```python
from build123d import *

# Parameters (mm, degrees)
EXTRUDE_1_DEPTH     = 6
EXTRUDE_2_DEPTH     = 20
EXTRUDE_4_DEPTH     = 6
SKETCH_5_R          = 7.25
EXTRUDE_5_DEPTH     = 14.8
SKETCH_6_R          = 4.25
SKETCH_6_R_2        = 1.25
EXTRUDE_6_DEPTH     = 10.2
EXTRUDE_7_DEPTH     = 76
CUT_EXTRUDE_1_DEPTH = 76


with BuildPart() as part:
    # 草图1 → 凸台-拉伸1 (new body)
    with BuildSketch(Plane(origin=(0, 0, 0), x_dir=(1, 0, 0), z_dir=(0, 1, 0))):
        with BuildLine():
            Line((-5, 0), (-5, -18))
            Line((-5, -18), (15, -18))
            Line((15, -18), (15, -88))
            Line((15, -88), (-10, -88))
            Line((-10, -88), (-10, -91))
            Line((-10, -91), (18, -91))
            Line((18, -91), (18, -15))
            Line((18, -15), (5, -15))
            Line((5, -15), (5, 0))
            ThreePointArc((5, 0), (0, 5), (-5, 0))
        make_face()
    extrude(amount=-EXTRUDE_1_DEPTH)

    # 草图2 → 凸台-拉伸2 (add, symmetric)
    with BuildSketch(Plane(origin=(0, 0, 0), x_dir=(1, 0, 0), z_dir=(0, 1, 0))):
        Polygon((-5, -18), (15, -18), (15, -88), (-10, -88), (-10, -91), (18, -91), (18, -15), (-5, -15), align=None)
    extrude(amount=EXTRUDE_2_DEPTH, both=True)

    # 草图4 → 凸台-拉伸4 (add)
    with BuildSketch(Plane.XZ.offset(6)):
        with BuildLine():
            ThreePointArc((-0.504732798, 8.734428762), (-0.823506466, 9.891100464), (-1.470958285, 10.901205517))
            ThreePointArc((-1.470958285, 10.901205517), (-1.726760313, 10.86362273), (-1.981608382, 10.820038273))
            ThreePointArc((-1.981608382, 10.820038273), (-2.283953757, 9.65896405), (-2.228374617, 8.460457882))
            ThreePointArc((-2.228374617, 8.460457882), (-2.708170263, 8.319303747), (-3.17911634, 8.150964378))
            ThreePointArc((-3.17911634, 8.150964378), (-3.839719327, 9.152518056), (-4.767622226, 9.913111434))
            ThreePointArc((-4.767622226, 9.913111434), (-4.999290692, 9.798320906), (-5.228197271, 9.678117239))
            ThreePointArc((-5.228197271, 9.678117239), (-5.156953143, 8.480440175), (-4.733735466, 7.357767973))
            ThreePointArc((-4.733735466, 7.357767973), (-5.146429214, 7.075257405), (-5.542305825, 6.76962681))
            ThreePointArc((-5.542305825, 6.76962681), (-6.480073708, 7.518023412), (-7.597598086, 7.954652936))
            ThreePointArc((-7.597598086, 7.954652936), (-7.782455665, 7.773891163), (-7.963013783, 7.588834659))
            ThreePointArc((-7.963013783, 7.588834659), (-7.525154025, 6.471791729), (-6.775725305, 5.53484847))
            ThreePointArc((-6.775725305, 5.53484847), (-7.080919818, 5.138635571), (-7.3629758, 4.725631002))
            ThreePointArc((-7.3629758, 4.725631002), (-8.486113324, 5.147612255), (-9.683868109, 5.217537585))
            ThreePointArc((-9.683868109, 5.217537585), (-9.803819655, 4.988498789), (-9.918355025, 4.756704069))
            ThreePointArc((-9.918355025, 4.756704069), (-9.1567404, 3.829639217), (-8.154459943, 3.170139435))
            ThreePointArc((-8.154459943, 3.170139435), (-8.322280653, 2.699008286), (-8.462906403, 2.219057507))
            ThreePointArc((-8.462906403, 2.219057507), (-9.661473042, 2.273316945), (-10.82221365, 1.969693302))
            ThreePointArc((-10.82221365, 1.969693302), (-10.86551747, 1.714797397), (-10.902818572, 1.458954141))
            ThreePointArc((-10.902818572, 1.458954141), (-9.892001226, 0.812614936), (-8.734979226, 0.495115065))
            ThreePointArc((-8.734979226, 0.495115065), (-8.748998674, -0.004816736), (-8.734428762, -0.504732798))
            ThreePointArc((-8.734428762, -0.504732798), (-9.891100464, -0.823506466), (-10.901205517, -1.470958285))
            ThreePointArc((-10.901205517, -1.470958285), (-10.86362273, -1.726760313), (-10.820038273, -1.981608382))
            ThreePointArc((-10.820038273, -1.981608382), (-9.65896405, -2.283953757), (-8.460457882, -2.228374617))
            ThreePointArc((-8.460457882, -2.228374617), (-8.319303747, -2.708170263), (-8.150964378, -3.17911634))
            ThreePointArc((-8.150964378, -3.17911634), (-9.152518056, -3.839719327), (-9.913111434, -4.767622226))
            ThreePointArc((-9.913111434, -4.767622226), (-9.798320906, -4.999290692), (-9.678117239, -5.228197271))
            ThreePointArc((-9.678117239, -5.228197271), (-8.480440175, -5.156953143), (-7.357767973, -4.733735466))
            ThreePointArc((-7.357767973, -4.733735466), (-7.075257405, -5.146429214), (-6.76962681, -5.542305825))
            ThreePointArc((-6.76962681, -5.542305825), (-7.518023412, -6.480073708), (-7.954652936, -7.597598086))
            ThreePointArc((-7.954652936, -7.597598086), (-7.773891163, -7.782455665), (-7.588834659, -7.963013783))
            ThreePointArc((-7.588834659, -7.963013783), (-6.471791729, -7.525154025), (-5.53484847, -6.775725305))
            ThreePointArc((-5.53484847, -6.775725305), (-5.138635571, -7.080919818), (-4.725631002, -7.3629758))
            ThreePointArc((-4.725631002, -7.3629758), (-5.147612255, -8.486113324), (-5.217537585, -9.683868109))
            ThreePointArc((-5.217537585, -9.683868109), (-4.988498789, -9.803819655), (-4.756704069, -9.918355025))
            ThreePointArc((-4.756704069, -9.918355025), (-3.829639217, -9.1567404), (-3.170139435, -8.154459943))
            ThreePointArc((-3.170139435, -8.154459943), (-2.699008286, -8.322280653), (-2.219057507, -8.462906403))
            ThreePointArc((-2.219057507, -8.462906403), (-2.273316945, -9.661473042), (-1.969693302, -10.82221365))
            ThreePointArc((-1.969693302, -10.82221365), (-1.714797397, -10.86551747), (-1.458954141, -10.902818572))
            ThreePointArc((-1.458954141, -10.902818572), (-0.812614936, -9.892001226), (-0.495115065, -8.734979226))
            ThreePointArc((-0.495115065, -8.734979226), (0.004816736, -8.748998674), (0.504732798, -8.734428762))
            ThreePointArc((0.504732798, -8.734428762), (0.823506466, -9.891100464), (1.470958285, -10.901205517))
            ThreePointArc((1.470958285, -10.901205517), (1.726760313, -10.86362273), (1.981608382, -10.820038273))
            ThreePointArc((1.981608382, -10.820038273), (2.283953757, -9.65896405), (2.228374617, -8.460457882))
            ThreePointArc((2.228374617, -8.460457882), (2.708170263, -8.319303747), (3.17911634, -8.150964378))
            ThreePointArc((3.17911634, -8.150964378), (3.839719327, -9.152518056), (4.767622226, -9.913111434))
            ThreePointArc((4.767622226, -9.913111434), (4.999290692, -9.798320906), (5.228197271, -9.678117239))
            ThreePointArc((5.228197271, -9.678117239), (5.156953143, -8.480440175), (4.733735466, -7.357767973))
            ThreePointArc((4.733735466, -7.357767973), (5.146429214, -7.075257405), (5.542305825, -6.76962681))
            ThreePointArc((5.542305825, -6.76962681), (6.480073708, -7.518023412), (7.597598086, -7.954652936))
            ThreePointArc((7.597598086, -7.954652936), (7.782455665, -7.773891163), (7.963013783, -7.588834659))
            ThreePointArc((7.963013783, -7.588834659), (7.525154025, -6.471791729), (6.775725305, -5.53484847))
            ThreePointArc((6.775725305, -5.53484847), (7.080919818, -5.138635571), (7.3629758, -4.725631002))
            ThreePointArc((7.3629758, -4.725631002), (8.486113324, -5.147612255), (9.683868109, -5.217537585))
            ThreePointArc((9.683868109, -5.217537585), (9.803819655, -4.988498789), (9.918355025, -4.756704069))
            ThreePointArc((9.918355025, -4.756704069), (9.1567404, -3.829639217), (8.154459943, -3.170139435))
            ThreePointArc((8.154459943, -3.170139435), (8.322280653, -2.699008286), (8.462906403, -2.219057507))
            ThreePointArc((8.462906403, -2.219057507), (9.661473042, -2.273316945), (10.82221365, -1.969693302))
            ThreePointArc((10.82221365, -1.969693302), (10.86551747, -1.714797397), (10.902818572, -1.458954141))
            ThreePointArc((10.902818572, -1.458954141), (9.892001226, -0.812614936), (8.734979226, -0.495115065))
            ThreePointArc((8.734979226, -0.495115065), (8.748998674, 0.004816736), (8.734428762, 0.504732798))
            ThreePointArc((8.734428762, 0.504732798), (9.891100464, 0.823506466), (10.901205517, 1.470958285))
            ThreePointArc((10.901205517, 1.470958285), (10.86362273, 1.726760313), (10.820038273, 1.981608382))
            ThreePointArc((10.820038273, 1.981608382), (9.65896405, 2.283953757), (8.460457882, 2.228374617))
            ThreePointArc((8.460457882, 2.228374617), (8.319303747, 2.708170263), (8.150964378, 3.17911634))
            ThreePointArc((8.150964378, 3.17911634), (9.152518056, 3.839719327), (9.913111434, 4.767622226))
            ThreePointArc((9.913111434, 4.767622226), (9.798320906, 4.999290692), (9.678117239, 5.228197271))
            ThreePointArc((9.678117239, 5.228197271), (8.480440175, 5.156953143), (7.357767973, 4.733735466))
            ThreePointArc((7.357767973, 4.733735466), (7.075257405, 5.146429214), (6.76962681, 5.542305825))
            ThreePointArc((6.76962681, 5.542305825), (7.518023412, 6.480073708), (7.954652936, 7.597598086))
            ThreePointArc((7.954652936, 7.597598086), (7.773891163, 7.782455665), (7.588834659, 7.963013783))
            ThreePointArc((7.588834659, 7.963013783), (6.471791729, 7.525154025), (5.53484847, 6.775725305))
            ThreePointArc((5.53484847, 6.775725305), (5.138635571, 7.080919818), (4.725631002, 7.3629758))
            ThreePointArc((4.725631002, 7.3629758), (5.147612255, 8.486113324), (5.217537585, 9.683868109))
            ThreePointArc((5.217537585, 9.683868109), (4.988498789, 9.803819655), (4.756704069, 9.918355025))
            ThreePointArc((4.756704069, 9.918355025), (3.829639217, 9.1567404), (3.170139435, 8.154459943))
            ThreePointArc((3.170139435, 8.154459943), (2.699008286, 8.322280653), (2.219057507, 8.462906403))
            ThreePointArc((2.219057507, 8.462906403), (2.273316945, 9.661473042), (1.969693302, 10.82221365))
            ThreePointArc((1.969693302, 10.82221365), (1.714797397, 10.86551747), (1.458954141, 10.902818572))
            ThreePointArc((1.458954141, 10.902818572), (0.812614936, 9.892001226), (0.495115065, 8.734979226))
            ThreePointArc((0.495115065, 8.734979226), (-0.004816736, 8.748998674), (-0.504732798, 8.734428762))
        make_face()
    extrude(amount=-EXTRUDE_4_DEPTH)

    # 草图5 → 凸台-拉伸5 (add)
    with BuildSketch(Plane(origin=(0, 0, 0), x_dir=(1, 0, 0), z_dir=(0, 1, 0))):
        with Locations(Location((0, 0, 0), (0, 0, 270))):
            Circle(SKETCH_5_R)
    extrude(amount=EXTRUDE_5_DEPTH)

    # 草图6 → 凸台-拉伸6 (add)
    with BuildSketch(Plane(origin=(0, 14.8, 0), x_dir=(1, 0, 0), z_dir=(0, 1, 0))):
        with Locations(Location((0, 0, 0), (0, 0, 270))):
            Circle(SKETCH_6_R)
        with Locations(Location((0, 0, 0), (0, 0, 270))):
            Circle(SKETCH_6_R_2, mode=Mode.SUBTRACT)
    extrude(amount=EXTRUDE_6_DEPTH)

    # 草图8 → 凸台-拉伸7 (add)
    with BuildSketch(Plane.XY.offset(91)):
        Polygon((-10, -20), (18, -10), (18, -20), align=None)
    extrude(amount=-EXTRUDE_7_DEPTH)

    # 草图9 → 切除-拉伸1 (cut)
    with BuildSketch(Plane(origin=(0, 0, 15), x_dir=(-1, 0, 0), z_dir=(0, 0, -1))):
        with BuildLine():
            Line((4.895011274, -19.977176364), (-17.212429644, -15.171210947))
            ThreePointArc((-17.212429644, -15.171210947), (-17.778597985, -14.821557633), (-18, -14.194034583))
            Line((-18, -14.194034583), (-18, -20))
            Line((-18, -20), (5.107440918, -20))
            ThreePointArc((5.107440918, -20), (5.000614807, -19.994277719), (4.895011274, -19.977176364))
        make_face()
    extrude(amount=-CUT_EXTRUDE_1_DEPTH, mode=Mode.SUBTRACT)


solid = part.part
```
Geometry check sheet. Reference: the model listing, model coordinates, mm. A direction names the side the tool comes from. Coordinates: 2 decimals unless noted, no trailing zeros. Write each loop counter-clockwise with the first axis right and the second up, starting at its lowest first coordinate (ties: lowest second). Pieces come first, ordered by that corner, then holes. Notation, with made-up numbers: M -3,80 L 34,80 A18 ccw 34,97 Z; hole C 67.5,51 d1. An arc over 180 degrees is marked long. Answer as a JSON object with one key per item and string values.
1. Go/stop test with flat-tipped pins: pin 1 Ø12 at (x, z) = (7, 57.5) entering from +Y; pin 2 Ø5 at (x, z) = (1, 80) entering from -Y; pin 3 Ø2.5 at (y, z) = (-0.5, 90) entering from -X. Record where each tip stops, or that it passes through.
Answers below:
{"pin 1": "stops at y = -11.79", "pin 2": "stops at y = -19.24", "pin 3": "stops at x = -10"}
2. Section check B-B, the plane y = 4. Enter the section's corners in (x, z).
Answers below:
{"outline": "M -10,88 L 15,88 L 15,18 L -5,18 L -5,15 L 18,15 L 18,91 L -10,91 Z; C 0,0 d14.5"}
3. Section check C-C, the plane z = 34. Enter the section's corners in (x, y).
Answers below:
{"outline": "M -10,-20 L -5.11,-20 A1 ccw -4.9,-19.98 L 17.21,-15.17 A1 ccw 18,-14.19 L 18,20 L 15,20 L 15,-11.07 Z"}
4. Section check D-D, the plane x = 12.75. Enter the section's corners in (y, z) (3 decimals), plus the area to 3 significant figures.
Answers below:
{"outline": "M -16.141,15 L 20,15 L 20,18 L -11.875,18 L -11.875,88 L 20,88 L 20,91 L -16.141,91 Z", "area": "515 mm²"}
5. Draft check along X on faces 4 (the cylindrical face through (5.16, -3.04, -8.5)), 5 (the cylindrical face through (9.14, -3.04, 3.83)), 6 (the flat face through (5, 1, 18)). Enter one of: released by +X, released by -X, zero draft, split by the parting line, or undercut.
Answers below:
{"face 4": "undercut", "face 5": "released by +X", "face 6": "zero draft"}
6. Section check A-A, the plane y = 17. Enter the section's corners in (x, z).
Answers below:
{"outline": "M -10,88 L 15,88 L 15,18 L -5,18 L -5,15 L 18,15 L 18,91 L -10,91 Z; C 0,0 d8.5; hole C 0,0 d2.5"}
7. Tool access check on faces 1 (the flat face through (5, -3, 12)), 2 (the cylindrical face through (-9.91, -3.04, 0.82)), 3 (the flat face through (-5, 1, 16)). Record the directions out of +Z, -Z, +X, -X, +Y, -Y that give a thin tool (end or side, any length) a straight path to the whole face; none if there is none.
Answers below:
{"face 1": "+X, +Y, -Y", "face 2": "-X, +Y, -Y", "face 3": "-X, +Y"}
8. Scan lines: L1, parallel to X at y = 20.75, z = 0; L2, parallel to Z at x = -5.5, y = 7; L3, parallel to Z at x = -8.5, y = -1. Record each from-to range of solid material in increasing order.
Answers below:
{"L1": "x = -4.25 to -1.25, 1.25 to 4.25", "L2": "z = -4.72 to 4.72, 88 to 91", "L3": "z = -5.16 to -3.36, -2.24 to 2.23, 3.35 to 5.15, 88 to 91"}
